```python
from build123d import *

# Parameters (mm, degrees)
F1_DEPTH = 2
F4_T     = -2


with BuildPart() as f1:
    # F0 (on Top) → F1 (new body)
    with BuildSketch(Plane.XY):
        Polygon((34.6410161514, -60), (34.6410161514, 60), (-69.2820323028, 0), align=None)
    extrude(amount=F1_DEPTH)

    # F2 (on face) → F3 section 0
    with BuildSketch(Plane.YZ.offset(34.6410161514), mode=Mode.PRIVATE) as f3_s0:
        Polygon((60, 2), (30, 42), (0, 42), (-30, 42), (-60, 2), align=None)
    loft([f3_s0.sketch, Vertex(-69.2820323028, 0, 2)])

    # F4
    f4_openings = [f1.faces().sort_by_distance(p)[0] for p in [
        (34.641016, 0, 18.604167),
    ]]
    offset(amount=F4_T, openings=f4_openings)


solid = f1.part
```
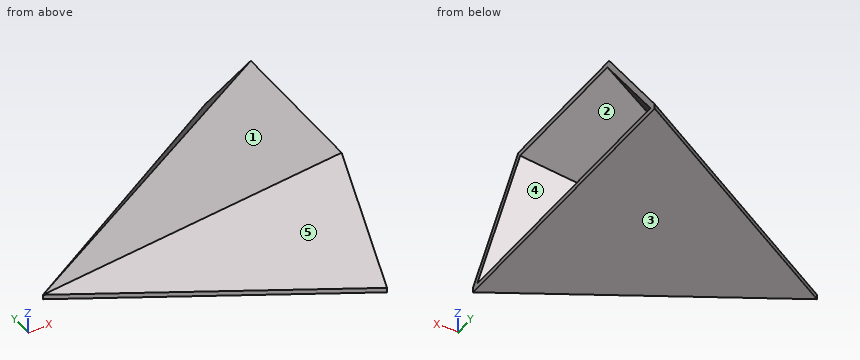
The model under review builds one solid part; all positions refer to its coordinate system, in mm. Face numbers are marked on the shaded views. A direction names the side the tool comes from. Round coordinates to 2 decimals unless told otherwise and drop trailing zeros. Loops run counter-clockwise (first coordinate to the right, second up) from the corner with the lowest first, then second, coordinate; pieces in that order, holes last. Notation, with made-up numbers: (51, 55) -> (61, 55) arc R29 cw to (61, 75) -> close; hole circle Ø4 at (-33.5, 9). An arc over 180 degrees is marked (long way). Answer as a JSON object with one key per item and string values. Group by question number.
1) We need section D-D on x = -43.5. Write out the cut boundary in (y, z), then the cut area to 3 significant figures.
2) We need section B-B on z = 21. Write out the cut boundary in (x, y).
3) We need section A-A on x = -4.5. Write out the cut boundary in (y, z).
4) We need section C-C on y = 49. Write out the cut boundary in (x, z).
5) For pin 1 Ø5 at (x, y) = (-20, 29.5) entering from +Z; pin 2 Ø3 at (x, y) = (23.5, 2.5) entering from -Z; pin 3 Ø12 at (x, y) = (-34, -4.5) entering from +Z; pin 4 Ø1.5 at (y, z) = (-21, 26) entering from -X, all flat-tipped, find the tip position at first contact; note any pin that passes through.
6) For the marked faces 4 and 5, list the 3-axis set-ups (+Z, -Z, +X, -X, +Y, -Y) from which the entire face can be reached by the end or side of a thin tool; tool diameter is ignored.
7) Mouldability with a two-part tool opening along Z and no side actions: class the marked faces 1, 2 and 3 as released by +Z, released by -Z, zero draft, split by the parting line, or undercut.
8) For line 1 (Z direction, x = 5, y = 33); line 2 (Y direction, x = 4.5, z = 7.5); line 3 (Z direction, x = 14, y = -30), list the stretches that pass through material, from the lowest coordinate up. Write a range as [from, to].
Result set:
{
 "1": {"outline": "(-14.89, 0) -> (14.89, 0) -> (14.89, 2) -> (7.44, 11.92) -> (-7.44, 11.92) -> (-14.89, 2) -> close; hole (-12.13, 2) -> (12.13, 2) -> (6.3, 9.78) -> (-6.3, 9.78) -> close", "area": "138 mm²"},
 "2": {"outline": "(-19.92, -14.25) -> (34.64, -45.75) -> (34.64, -43) -> (-14.35, -14.71) -> (-14.35, 14.71) -> (34.64, 43) -> (34.64, 45.75) -> (-19.92, 14.25) -> close"},
 "3": {"outline": "(-37.4, 0) -> (37.4, 0) -> (37.4, 2) -> (18.7, 26.93) -> (-18.7, 26.93) -> (-37.4, 2) -> close; hole (-34.65, 2) -> (34.65, 2) -> (17.55, 24.79) -> (-17.55, 24.79) -> close"},
 "4": {"outline": "(15.59, 0) -> (34.64, 0) -> (34.64, 2) -> (20.36, 2) -> (34.64, 12.99) -> (34.64, 16.67) -> (15.59, 2) -> close"},
 "5": {"pin 1": "z = 4.45", "pin 2": "z = 0", "pin 3": "z = 17.89", "pin 4": "x = -3.36"},
 "6": {"face 4": "+X", "face 5": "+Z, -X, -Y"},
 "7": {"face 1": "released by +Z", "face 2": "undercut", "face 3": "released by -Z"},
 "8": {"line 1": "[0, 2], [11.51, 15.18]", "line 2": "[-38.47, -35.72], [35.72, 38.47]", "line 3": "[0, 2], [22.44, 26.11]"}
}
